Geometry: see drawing. Coordinates: mm, zero at the bounding-box minimum. A direction names the side the tool comes from. Round coordinates to 2 decimals unless told otherwise and drop trailing zeros. Loops run counter-clockwise (first coordinate to the right, second up) from the corner with the lowest first, then second, coordinate; pieces in that order, holes last. Notation, with made-up numbers: (42, -22.5) -> (96, -22.5) arc R16 cw to (96, -14.5) -> close; hole circle Ø5 at (7, -2.75). An arc over 180 degrees is marked (long way). Answer in a Markdown table with one row per item.
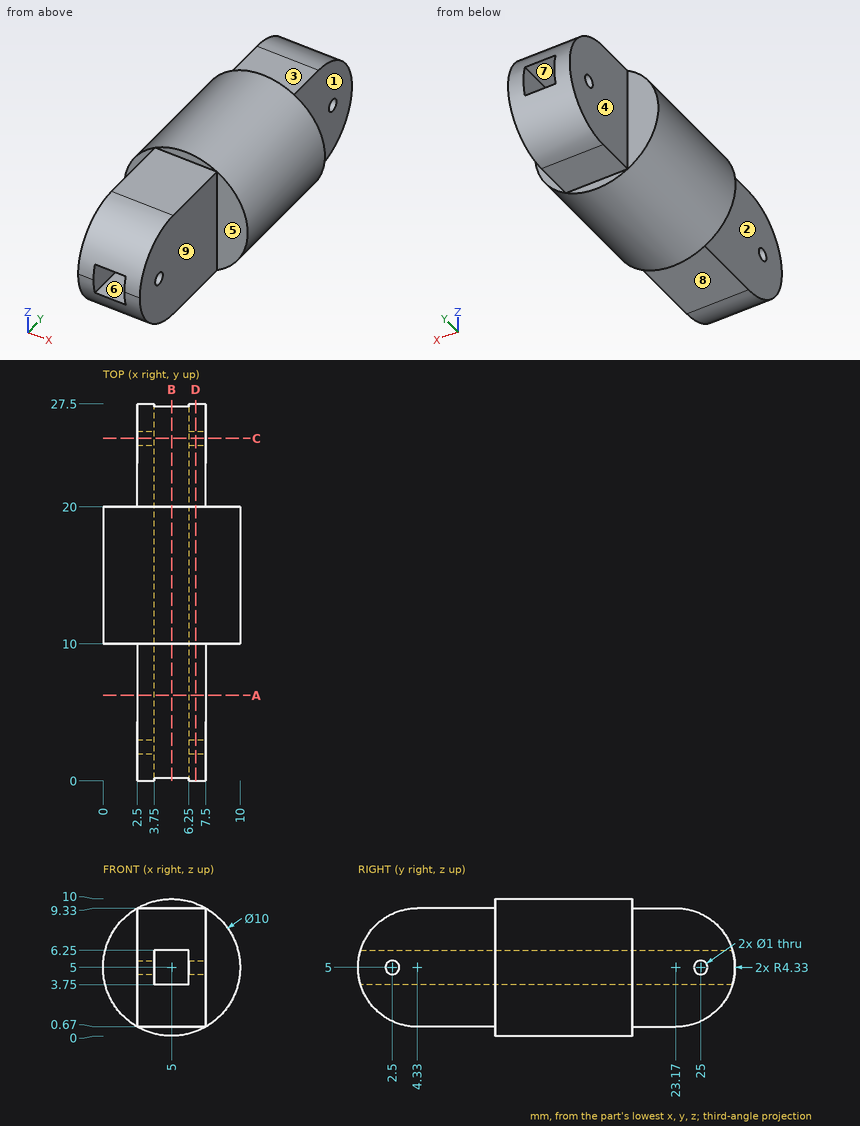
Item 1: Ray query, L1, parallel to Y at x = 6.7, z = 5; L2, parallel to X at y = 3.75, z = 6; L3, parallel to Y at x = 7, z = 0.5. Return the intervals inside material, ascending.
Ans:
| item | result |
|---|---|
| L1 | 0 to 2, 3 to 24.5, 25.5 to 27.5 |
| L2 | 2.5 to 3.75, 6.25 to 7.5 |
| L3 | 10 to 20 |
Item 2: Section query B-B, the plane x = 5. Output: boundary loops of the cut face in (y, z).
Ans:
| item | result |
|---|---|
| outline | (0.18, 3.75) arc R4.33 ccw to (4.33, 0.67) -> (10, 0.67) -> (10, 0) -> (20, 0) -> (20, 0.67) -> (23.17, 0.67) arc R4.33 ccw to (27.32, 3.75) -> close; (0.18, 6.25) -> (27.32, 6.25) arc R4.33 ccw to (23.17, 9.33) -> (20, 9.33) -> (20, 10) -> (10, 10) -> (10, 9.33) -> (4.33, 9.33) arc R4.33 ccw to start |
Item 3: Section query D-D, the plane x = 6.75. Output: boundary loops of the cut face in (y, z), and give its area (3 significant figures).
Ans:
| item | result |
|---|---|
| outline | (4.33, 0.67) -> (10, 0.67) -> (10, 0.32) -> (20, 0.32) -> (20, 0.67) -> (23.17, 0.67) arc R4.33 ccw to (23.17, 9.33) -> (20, 9.33) -> (20, 9.68) -> (10, 9.68) -> (10, 9.33) -> (4.33, 9.33) arc R4.33 ccw to start; hole circle Ø1 at (2.5, 5); hole circle Ø1 at (25, 5) |
| area | 228 mm2 |
Item 4: Section query C-C, the plane y = 25. Output: boundary loops of the cut face in (x, z), and give its area (3 significant figures).
Ans:
| item | result |
|---|---|
| outline | (2.5, 1.08) -> (7.5, 1.08) -> (7.5, 4.5) -> (6.25, 4.5) -> (6.25, 3.75) -> (3.75, 3.75) -> (3.75, 4.5) -> (2.5, 4.5) -> close; (2.5, 5.5) -> (3.75, 5.5) -> (3.75, 6.25) -> (6.25, 6.25) -> (6.25, 5.5) -> (7.5, 5.5) -> (7.5, 8.92) -> (2.5, 8.92) -> close |
| area | 30.5 mm2 |
Item 5: Set-up query: the marked faces 1, 2, 3, 4 and 5. Return all of +Z, -Z, +X, -X, +Y, -Y with unobstructed straight access to the full face (end or side cutting, diameter ignored); none if empty.
Ans:
| item | result |
|---|---|
| face 1 | +Z, -Z, +X, +Y |
| face 2 | +Z, -Z, -X, -Y |
| face 3 | +Z, +X, -X, +Y |
| face 4 | +Z, -Z, -X, +Y |
| face 5 | +Z, -Z, +X, -Y |
Item 6: Mould query, pull axis X, two halves, no side actions, for the marked faces 6, 7, 8 and 9. Classes: released by +X, released by -X, zero draft, split by the parting line, or undercut.
Ans:
| item | result |
|---|---|
| face 6 | undercut |
| face 7 | undercut |
| face 8 | zero draft |
| face 9 | released by +X |
Item 7: Section query A-A, the plane y = 6.25. Output: boundary loops of the cut face in (x, z).
Ans:
| item | result |
|---|---|
| outline | (2.5, 0.67) -> (7.5, 0.67) -> (7.5, 9.33) -> (2.5, 9.33) -> close; hole (3.75, 3.75) -> (6.25, 3.75) -> (6.25, 6.25) -> (3.75, 6.25) -> close |
Item 8: First-contact query: P1, Ø1.3, axis at y = 25, z = 5, coming from the +X side; P2, Ø3, axis at x = 8.5, z = 3, coming from the -Y side; P3, Ø4, axis at y = 20.5, z = 8, coming from the +X side; P4, Ø0.6, axis at y = 2.5, z = 5, coming from the +X side. Flat tips, straight axial feed; report the tip coordinate or a pass-through.
Ans:
| item | result |
|---|---|
| P1 | x = 7.5 |
| P2 | y = 0.09 |
| P3 | x = 9.89 |
| P4 | through |
